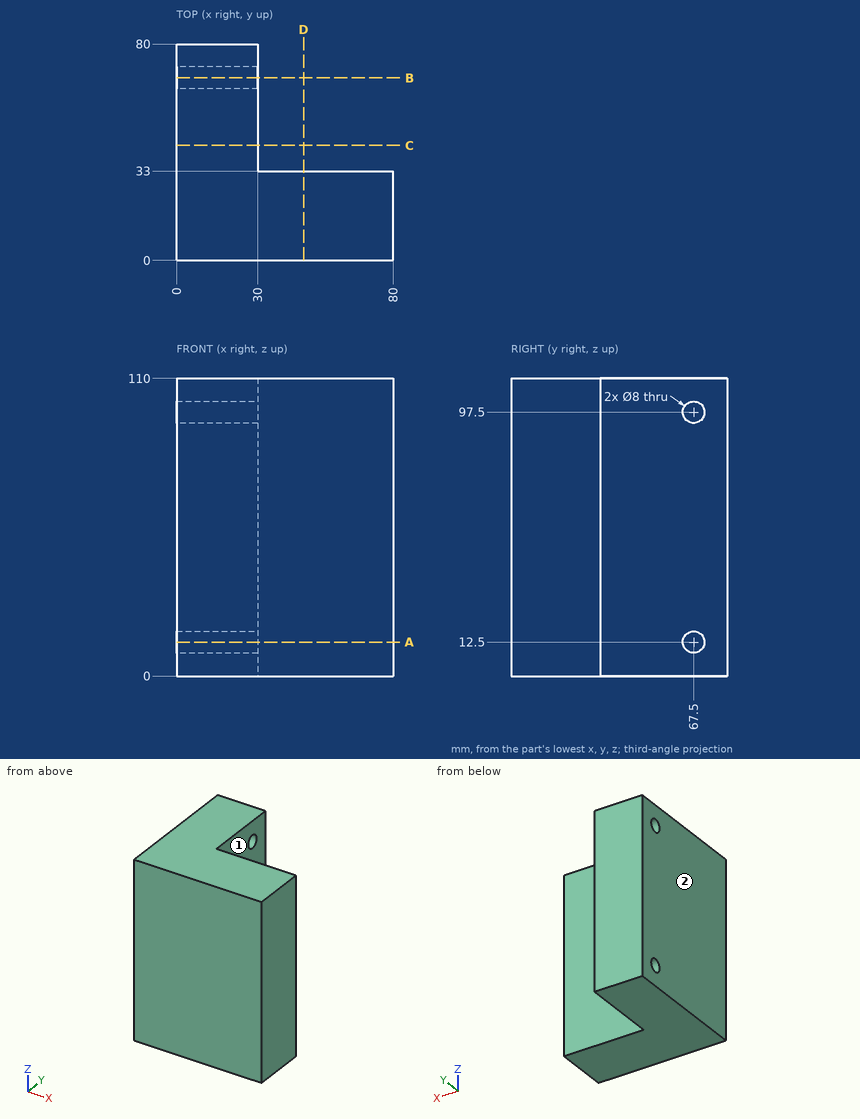
Answer from the drawing. Dimensions are ordinates in mm from the lowest x, y and z of the part. A direction names the side the tool comes from. Give positions to 0.01 mm unless a question says otherwise; leave off trailing zeros. Order: outer loops, then holes, each group sorted by start corner. A loop starts at its lowest first (then second) coordinate and runs counter-clockwise, first axis right, second up.
(1) Find section A-A (z = 12.5). Give the vertices of the cut face in (x, y), plus the area to 3 significant figures.
(2) Find section C-C (y = 42.5). Give the vertices of the cut face in (x, z).
(3) Find section B-B (y = 67.5). Give the vertices of the cut face in (x, z), plus the area to 3 significant figures.
(4) For the marked faces 1 and 2, determine the directions among +Z, -Z, +X, -X, +Y, -Y from which every point of the face is accessible in a straight line to the end or side of a thin tool.
(5) Find section D-D (x = 47). Give the vertices of the cut face in (y, z).
(6) Straight lines are drawn through the part: L1, parallel to Z at x = 9, y = 67; L2, parallel to Y at x = 20, z = 97; L3, parallel to Y at x = 76.5, z = 29.5. For each, find the intervals that lie inside material, in ascending order.
(7) Given pin 1 (12 mm diameter, centred on x = 66.5, z = 73, fed in from +Y); pin 2 (14 mm diameter, centred on y = 48, z = 34.5, fed in from +X), each flat-ended and moving along its own axis, determine where each tip first touches the part or whether it passes through.
Result sheet:
1. outline: (0, 0) - (80, 0) - (80, 33) - (30, 33) - (30, 63.5) - (0, 63.5) - close; (0, 71.5) - (30, 71.5) - (30, 80) - (0, 80) - close
1. area: 3,810 mm2
2. outline: (0, 0) - (30, 0) - (30, 110) - (0, 110) - close
3. outline: (0, 0) - (30, 0) - (30, 8.5) - (0, 8.5) - close; (0, 16.5) - (30, 16.5) - (30, 93.5) - (0, 93.5) - close; (0, 101.5) - (30, 101.5) - (30, 110) - (0, 110) - close
3. area: 2,820 mm2
4. face 1: +Z, -Z, +X, +Y
4. face 2: +Z, -Z, -X, +Y, -Y
5. outline: (0, 0) - (33, 0) - (33, 110) - (0, 110) - close
6. L1: z = 0 to 8.53, 16.47 to 93.53, 101.47 to 110
6. L2: y = 0 to 63.53, 71.47 to 80
6. L3: y = 0 to 33
7. pin 1: stops at y = 33
7. pin 2: stops at x = 30
